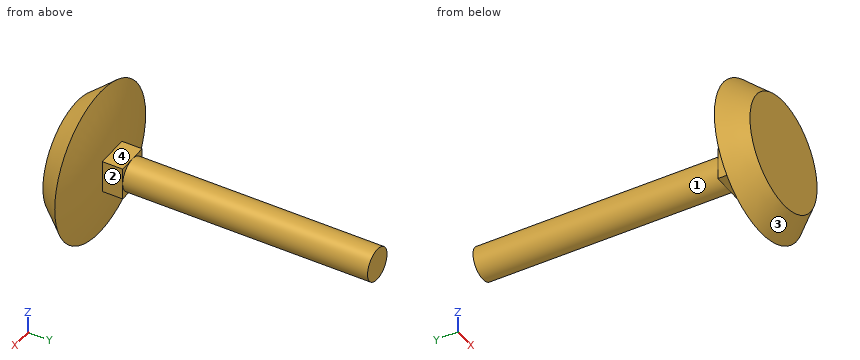
from build123d import *

# Parameters (mm, degrees)
EXTRUDE1_DEPTH = 4.6736


with BuildPart() as part:
    # Sketch1 → Revolve1 (revolve)
    with BuildSketch(Plane.XY):
        with BuildLine():
            Line((152.4, 939.2412), (152.4, 853.44))
            Line((152.4, 853.44), (136.271, 853.44))
            Line((136.271, 853.44), (130.556, 860.202760353))
            ThreePointArc((130.556, 860.202760353), (139.032835502, 862.449078304), (147.726400001, 863.6))
            Line((147.726400001, 863.6), (147.726400001, 939.2412))
            Line((147.726400001, 939.2412), (152.4, 939.2412))
        make_face()
    revolve(axis=Axis((152.4, 939.2412, 0), (0, -1, 0)))

    # Sketch2 → Extrude1 (add, symmetric)
    with BuildSketch(Plane.XY):
        Polygon((157.073600006, 863.600000001), (157.073599999, 869.3912), (147.726400001, 869.3912), (147.726400001, 863.6), align=None)
    extrude(amount=EXTRUDE1_DEPTH, both=True)


solid = part.part
Check sheet for the modelled part. Datum: model origin and axes. Units: mm. Face numbers are marked on the shaded views. A direction names the side the tool comes from. Round coordinates to 2 decimals unless told otherwise and drop trailing zeros. Loops run counter-clockwise (first coordinate to the right, second up) from the corner with the lowest first, then second, coordinate; pieces in that order, holes last. Notation, with made-up numbers: M 52,34.5 L 101,34.5 A24 cw 101,62.5 Z; hole C 55,74 d7. An arc over 180 degrees is marked long. One line per question, with ' | ' between items. Start each with the question number.
Item 1: Section check A-A (y = 867). Record the boundary of the cut face in (x, z).
Item 2: Gauge pin test, flat ends, axial feed: pin 1 Ø4.5 at (x, y) = (150.5, 867) entering from -Z; pin 2 Ø10 at (y, z) = (919, 4) entering from -X; pin 3 Ø1.5 at (y, z) = (879, 4.5) entering from +X; pin 4 Ø3 at (x, y) = (160.5, 906) entering from +Z. Record the tip position at first contact, or that the pin passes through.
Item 3: Section check B-B (y = 890). Record the boundary of the cut face in (x, z).
Item 4: Scan lines: probe 1 along Y at (x, z) = (146, 18); probe 2 along X at (y, z) = (889.5, -4); probe 3 along Z at (x, y) = (149.5, 917.5). Record each from-to range of solid material in increasing order.
Item 5: Set-up check for the marked faces 1, 2, 3 and 4: record each of +Z, -Z, +X, -X, +Y, -Y from which the full face is reachable in a straight line by a thin tool's end or side.
Worked out:
1) outline: M 147.73,-4.67 L 157.07,-4.67 L 157.07,4.67 L 147.73,4.67 Z
2) pin 1: z = -4.67 | pin 2: x = 147.73 | pin 3: x = 155.19 | pin 4: through
3) outline: C 152.4,0 d9.35
4) probe 1: 856.96 to 861.06 | probe 2: 149.98 to 154.82 | probe 3: -3.67 to 3.67
5) face 1: +Y | face 2: +Z, -Z, +X, +Y | face 3: -Y | face 4: +Z, +X, -X, +Y
